Autodesk Inventor part; units mm, degrees
ref_plane "YZ Plane" through (0, 0, 0) normal (1, 0, 0) x (0, 1, 0)
ref_plane "XZ Plane" through (0, 0, 0) normal (0, 1, 0) x (-1, 0, 0)
ref_plane "XY Plane" through (0, 0, 0) normal (0, 0, 1) x (1, 0, 0)
sketch "Skizze1" plane through (0, 0, 0) normal (0, 0, 1) x (1, 0, 0)
  circle A0 centre (0, 0) radius 10
  dimension "d0" = 20
extrude "Extrusion1" add sketch "Skizze1" along normal blind 170
sketch "Skizze5" plane through (0, 0, 0) normal (0, 1, 0) x (-1, 0, 0)
  circle A0 centre (0, 100) radius 5
  line L0 (0, -21) -> (0, 126)
  line L1 (7, 0) -> (-7, 0)
  point P0 (0, 0)
  dimension "d11" = 10
  dimension "d12" = 0
  dimension "d13" = 100
extrude "Extrusion4" add sketch "Skizze5" against normal blind 70
sketch "Skizze6" plane through (0, 0, 0) normal (1, 0, 0) x (0, 1, 0)
  line L0 (10, 170) -> (-10, 170)
  line L1 (0, 170) -> (0, 70)
  circle A0 centre (0, 70) radius 5
  point P0 (0, 0)
  dimension "d17" = 100
  dimension "d18" = 10
extrude "Extrusion5" add sketch "Skizze6" along normal blind 70
sketch "Skizze7" plane through (0, 0, 0) normal (0, 0, -1) x (-1, 0, 0)
  circle A0 centre (0, 0) radius 8.5
extrude "Extrusion6" cut sketch "Skizze7" against normal blind 60
thread "Gewinde1"
thread "Gewinde2"
chamfer "Fasen1" distance 1 angle 45 1 edges at (5, -70, 100)
chamfer "Fasen2" distance 1 angle 45 1 edges at (70, -5, 70)
sketch "Skizze8" plane through (0, 0, 170) normal (0, 0, 1) x (1, 0, 0)
  point P0 (0, 0)
hole "Bohrung1" at (0, 0, 170) direction (0, 0, -1) diameter 6.647 depth 22.2 tip angle 118
properties part number "HTW-000681" material "Edelstahl"
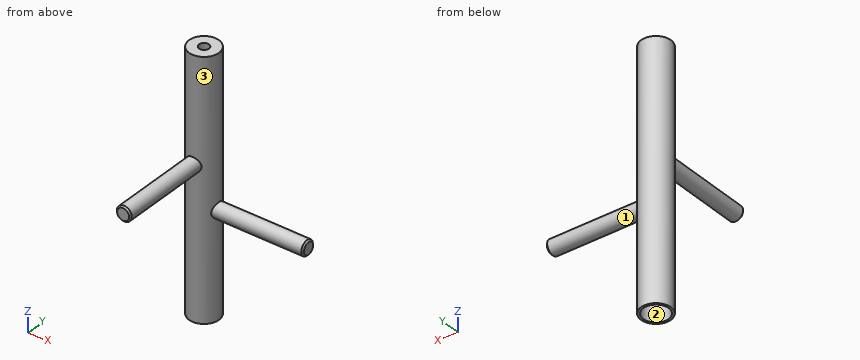
For this review, take the finished solid that the model builds, in its own axes (mm). Face numbers are marked on the shaded views. Coordinates: 2 decimals unless noted, no trailing zeros. Write each loop counter-clockwise with the first axis right and the second up, starting at its lowest first coordinate (ties: lowest second). Pieces come first, ordered by that corner, then holes. Notation, with made-up numbers: (50.25, 9) - (61.25, 9) arc R18 cw to (61.25, 35) - close; hole circle Ø8 at (-9, 49). An arc over 180 degrees is marked (long way). Put each result on its own line as item: value.
1. Wall thickness on probe 1 along Y at (x, z) = (0, 155); probe 2 along Y at (x, z) = (0, 24.5); probe 3 along Y at (x, z) = (-5, 156): over which ranges is each line inside the solid? List them lowest first.
Values found:
probe 1: -10 to -3.32, 3.32 to 10
probe 2: -10 to -8.5, 8.5 to 10
probe 3: -8.66 to 8.66
2. Add section C-C, the plane y = -34.5. Give the boundary of the cut face in (x, z).
Values found:
outline: circle Ø10 at (0, 100)
3. For pin 1 (8 mm diameter, centred on x = 11.5, z = 93.5, fed in from +Y); pin 2 (4 mm diameter, centred on x = 6, y = -39, fed in from -Z); pin 3 (8 mm diameter, centred on x = 16.5, y = -12.5, fed in from +Z); pin 4 (12 mm diameter, centred on y = 1, z = 124, fed in from +X), all flat-tipped, find the tip position at first contact; note any pin that passes through.
Values found:
pin 1: y = 6.61
pin 2: z = 97
pin 3: through
pin 4: x = 10
4. Mouldability with a two-part tool opening along X and no side actions: class the marked faces 1, 2 and 3 as released by +X, released by -X, zero draft, split by the parting line, or undercut.
Values found:
face 1: zero draft
face 2: undercut
face 3: split by the parting line
5. Add section B-B, the plane z = 70. Give the boundary of the cut face in (x, y), then the cut area to 4 significant figures.
Values found:
outline: (8.66, -5) - (69, -5) - (70, -4) - (70, 4) - (69, 5) - (8.66, 5) arc R10 ccw (long way) to start
area: 917.5 mm²
6. Add section A-A, the plane z = 28.5. Give the boundary of the cut face in (x, y), then the cut area to 3 significant figures.
Values found:
outline: circle Ø20 at (0, 0); hole circle Ø17 at (0, 0)
area: 87.2 mm²
7. Add section D-D, the plane x = 56.5. Give the boundary of the cut face in (y, z).
Values found:
outline: circle Ø10 at (0, 70)
